Work out the finished part from the listing and answer in its coordinate system (mm). Round coordinates to 2 decimals unless told otherwise and drop trailing zeros. Write each loop counter-clockwise with the first axis right and the second up, starting at its lowest first coordinate (ties: lowest second). Pieces come first, ordered by that corner, then holes. Notation, with made-up numbers: M 8,0.5 L 17,0.5 A23 ccw 17,15.5 Z; hole C 8,-23.5 d9. An arc over 180 degrees is marked long. Answer in a Markdown table with one row per item.
```python
from build123d import *

# Parameters (mm, degrees)
SKETCH_1_W          = 136
SKETCH_1_H          = 88
EXTRUDE_1_DEPTH     = 2
SKETCH_2_R          = 1.6
SKETCH_2_W          = 4
SKETCH_2_H          = 10
SKETCH_2_H_2        = 20
CUT_EXTRUDE_1_DEPTH = 2
SKETCH_5_R          = 1.6
CUT_EXTRUDE_2_DEPTH = 10
SKETCH_6_R          = 1.6
CUT_EXTRUDE_3_DEPTH = 10
SKETCH_10_R         = 1.6
CUT_EXTRUDE_4_DEPTH = 10
SKETCH_11_R         = 4
EXTRUDE_3_DEPTH     = 200
SKETCH_13_W         = 20
SKETCH_13_H         = 2
CUT_EXTRUDE_5_DEPTH = 2
CUT_EXTRUDE_6_DEPTH = 10
SKETCH_15_W         = 5
SKETCH_15_H         = 15
CUT_EXTRUDE_7_DEPTH = 5
SKETCH_16_R         = 1.6
CUT_EXTRUDE_8_DEPTH = 10


with BuildPart() as part:
    # 草图1 → 凸台-拉伸1 (new body)
    with BuildSketch(Plane(origin=(0, 0, 0), x_dir=(1, 0, 0), z_dir=(0, 1, 0))):
        with Locations((68, -44)):
            Rectangle(SKETCH_1_W, SKETCH_1_H)
    extrude(amount=EXTRUDE_1_DEPTH)

    # 草图2 → 切除-拉伸1 (cut)
    with BuildSketch(Plane(origin=(0, 2, 0), x_dir=(1, 0, 0), z_dir=(0, 1, 0))):
        with Locations(Location((4, -29, 0), (0, 0, 270))):
            Circle(SKETCH_2_R)
        with Locations(Location((4, -9, 0), (0, 0, 270))):
            Circle(SKETCH_2_R)
        with Locations(Location((132, -9, 0), (0, 0, 90))):
            Circle(SKETCH_2_R)
        with Locations(Location((132, -29, 0), (0, 0, 90))):
            Circle(SKETCH_2_R)
        with Locations(Location((132, -59, 0), (0, 0, 270))):
            Circle(SKETCH_2_R)
        with Locations(Location((132, -79, 0), (0, 0, 270))):
            Circle(SKETCH_2_R)
        with Locations(Location((4, -79, 0), (0, 0, 90))):
            Circle(SKETCH_2_R)
        with Locations(Location((4, -59, 0), (0, 0, 90))):
            Circle(SKETCH_2_R)
        Polygon((4, -44), (4, -34), (8, -34), (8, -44), (8, -54), (4, -54), align=None)
        with Locations((6, -19)):
            Rectangle(SKETCH_2_W, SKETCH_2_H)
        with Locations((130, -19)):
            Rectangle(SKETCH_2_W, SKETCH_2_H)
        with Locations((130, -44)):
            Rectangle(SKETCH_2_W, SKETCH_2_H_2)
        with Locations((130, -69)):
            Rectangle(SKETCH_2_W, SKETCH_2_H)
        with Locations((6, -69)):
            Rectangle(SKETCH_2_W, SKETCH_2_H)
    extrude(amount=-CUT_EXTRUDE_1_DEPTH, mode=Mode.SUBTRACT)

    # 草图5 → 切除-拉伸2 (cut)
    with BuildSketch(Plane(origin=(0, 2, 0), x_dir=(1, 0, 0), z_dir=(0, 1, 0))):
        with Locations(Location((12, -28, 0), (0, 0, 270))):
            Circle(SKETCH_5_R)
        with Locations(Location((12, -60, 0), (0, 0, 270))):
            Circle(SKETCH_5_R)
        with Locations(Location((124, -60, 0), (0, 0, 270))):
            Circle(SKETCH_5_R)
        with Locations(Location((124, -28, 0), (0, 0, 270))):
            Circle(SKETCH_5_R)
        with Locations(Location((12, -79, 0), (0, 0, 270))):
            Circle(SKETCH_5_R)
        with Locations(Location((12, -84, 0), (0, 0, 270))):
            Circle(SKETCH_5_R)
        with Locations(Location((12, -9, 0), (0, 0, 270))):
            Circle(SKETCH_5_R)
        with Locations(Location((12, -4, 0), (0, 0, 270))):
            Circle(SKETCH_5_R)
        with Locations(Location((124, -84, 0), (0, 0, 270))):
            Circle(SKETCH_5_R)
        with Locations(Location((124, -79, 0), (0, 0, 270))):
            Circle(SKETCH_5_R)
        with Locations(Location((124, -4, 0), (0, 0, 270))):
            Circle(SKETCH_5_R)
        with Locations(Location((124, -9, 0), (0, 0, 270))):
            Circle(SKETCH_5_R)
    extrude(amount=-CUT_EXTRUDE_2_DEPTH, mode=Mode.SUBTRACT)

    # 草图6 → 切除-拉伸3 (cut)
    with BuildSketch(Plane(origin=(0, 2, 0), x_dir=(1, 0, 0), z_dir=(0, 1, 0))):
        with Locations(Location((68, -35, 0), (0, 0, 270))):
            Circle(SKETCH_6_R)
        with Locations(Location((68, -53, 0), (0, 0, 270))):
            Circle(SKETCH_6_R)
        with Locations(Location((77, -44, 0), (0, 0, 270))):
            Circle(SKETCH_6_R)
        with Locations(Location((59, -44, 0), (0, 0, 270))):
            Circle(SKETCH_6_R)
    extrude(amount=-CUT_EXTRUDE_3_DEPTH, mode=Mode.SUBTRACT)

    # 草图10 → 切除-拉伸4 (cut)
    with BuildSketch(Plane(origin=(0, 2, 0), x_dir=(1, 0, 0), z_dir=(0, 1, 0))):
        with Locations(Location((21, -85, 0), (0, 0, 270))):
            Circle(SKETCH_10_R)
        with Locations(Location((21, -61, 0), (0, 0, 270))):
            Circle(SKETCH_10_R)
        with Locations(Location((115, -61, 0), (0, 0, 270))):
            Circle(SKETCH_10_R)
        with Locations(Location((115, -85, 0), (0, 0, 270))):
            Circle(SKETCH_10_R)
    extrude(amount=-CUT_EXTRUDE_4_DEPTH, mode=Mode.SUBTRACT)

    # 草图11 → 凸台-拉伸3 (add)
    with BuildSketch(Plane.XZ):
        with Locations(Location((68, 44, 0), (0, 0, 270))):
            Circle(SKETCH_11_R)
    extrude(amount=-EXTRUDE_3_DEPTH)

    # 草图13 → 切除-拉伸5 (cut)
    with BuildSketch(Plane(origin=(0, 2, 0), x_dir=(1, 0, 0), z_dir=(0, 1, 0))):
        with Locations((43, -4)):
            Rectangle(SKETCH_13_W, SKETCH_13_H)
        with Locations((43, -31)):
            Rectangle(SKETCH_13_W, SKETCH_13_H)
        with Locations((93, -31)):
            Rectangle(SKETCH_13_W, SKETCH_13_H)
        with Locations((93, -4)):
            Rectangle(SKETCH_13_W, SKETCH_13_H)
    extrude(amount=-CUT_EXTRUDE_5_DEPTH, mode=Mode.SUBTRACT)

    # 草图14 → 切除-拉伸6 (cut)
    with BuildSketch(Plane(origin=(0, 2, 0), x_dir=(1, 0, 0), z_dir=(0, 1, 0))):
        Polygon((13, -44), (13, -34), (30, -34), (30, -54), (13, -54), align=None)
        Polygon((106, -34), (106, -54), (123, -54), (123, -44), (123, -34), align=None)
    extrude(amount=-CUT_EXTRUDE_6_DEPTH, mode=Mode.SUBTRACT)

    # 草图15 → 切除-拉伸7 (cut)
    with BuildSketch(Plane(origin=(0, 2, 0), x_dir=(1, 0, 0), z_dir=(0, 1, 0))):
        with Locations((68, -73)):
            Rectangle(SKETCH_15_W, SKETCH_15_H)
        with Locations((80.5, -73)):
            Rectangle(SKETCH_15_W, SKETCH_15_H)
        with Locations((93, -73)):
            Rectangle(SKETCH_15_W, SKETCH_15_H)
        with Locations((105.5, -73)):
            Rectangle(SKETCH_15_W, SKETCH_15_H)
        with Locations((55.5, -73)):
            Rectangle(SKETCH_15_W, SKETCH_15_H)
        with Locations((43, -73)):
            Rectangle(SKETCH_15_W, SKETCH_15_H)
        with Locations((30.5, -73)):
            Rectangle(SKETCH_15_W, SKETCH_15_H)
    extrude(amount=-CUT_EXTRUDE_7_DEPTH, mode=Mode.SUBTRACT)

    # 草图16 → 切除-拉伸8 (cut)
    with BuildSketch(Plane.XZ):
        with Locations(Location((88, 15, 0), (0, 0, 270))):
            Circle(SKETCH_16_R)
        with Locations(Location((48, 15, 0), (0, 0, 270))):
            Circle(SKETCH_16_R)
        with Locations(Location((98, 15, 0), (0, 0, 270))):
            Circle(SKETCH_16_R)
        with Locations(Location((38, 15, 0), (0, 0, 270))):
            Circle(SKETCH_16_R)
    extrude(amount=-CUT_EXTRUDE_8_DEPTH, mode=Mode.SUBTRACT)


solid = part.part
```
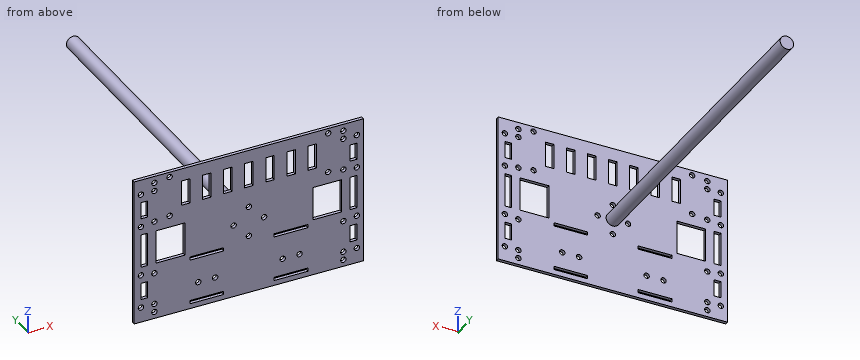
1. The part is cut by section B-B (y = 165.5). Determine the outline of the cut face in (x, z).
Calculated:
| item | result |
|---|---|
| outline | C 68,44 d8 |
2. Consider line 1 along Z through (x, y) = (68, 1.25); line 2 along X through (y, z) = (1.2, 35); line 3 along Z through (x, y) = (98, 0.75). Determine where each line is inside the solid, lowest interval first. Write a range as from..to.
Calculated:
| item | result |
|---|---|
| line 1 | z = 0..33.4, 36.6..51.4, 54.6..65.5, 80.5..88 |
| line 2 | x = 0..4, 8..13, 30..66.4, 69.6..106, 123..128, 132..136 |
| line 3 | z = 0..3, 5..13.4, 16.6..30, 32..88 |
3. The part is cut by section A-A (z = 21). Determine the outline of the cut face in (x, y).
Calculated:
| item | result |
|---|---|
| outline | M 0,0 L 4,0 L 4,2 L 0,2 Z; M 8,0 L 128,0 L 128,2 L 8,2 Z; M 132,0 L 136,0 L 136,2 L 132,2 Z |
4. Given pin 1 (12 mm diameter, centred on x = 69.5, z = 30.5, fed in from +Y); pin 2 (6 mm diameter, centred on y = 27.5, z = 38, fed in from +X); pin 3 (1 mm diameter, centred on y = 109.5, z = 42.5, fed in from +X), each flat-ended and moving along its own axis, determine where each tip first touches the part or whether it passes through.
Calculated:
| item | result |
|---|---|
| pin 1 | stops at y = 2 |
| pin 2 | stops at x = 70.65 |
| pin 3 | stops at x = 71.87 |
